Can you work these out from the model? Positions are in its coordinate system, mm. Face numbers are marked on the shaded views. A direction names the side the tool comes from. Coordinates: 2 decimals unless noted, no trailing zeros. Write each loop counter-clockwise with the first axis right and the second up, starting at its lowest first coordinate (ties: lowest second). Pieces come first, ordered by that corner, then holes.
Autodesk Inventor part; units mm, degrees
ref_plane "Work Plane1" through (13.2035, 0, 0) normal (0, 0, 1) x (-1, 0, 0)
ref_plane "YZ Plane" through (0, 0, 0) normal (1, 0, 0) x (0, 1, 0)
ref_plane "XZ Plane" through (0, 0, 0) normal (0, 1, 0) x (-1, 0, 0)
sketch "Skizze1" plane through (0, 0, 0) normal (1, 0, 0) x (0, 1, 0)
  line L0 (2.3094, -4) -> (-2.3094, -4)
  line L1 (-2.3094, -4) -> (-4.6188, 0)
  line L2 (-4.6188, 0) -> (-2.3094, 4)
  line L3 (-2.3094, 4) -> (2.3094, 4)
  line L4 (2.3094, 4) -> (4.6188, 0)
  line L5 (4.6188, 0) -> (2.3094, -4)
  point P0 (0, 0)
  point P1 (0, 0)
  dimension "d0" = 9.2376
extrude "Körper" add sketch "Skizze1" along normal blind 2.45
sketch "Skizze2" plane through (2.45, 0, 0) normal (1, 0, 0) x (0, 0, -1)
  circle A0 centre (0, 0) radius 3.45
  dimension "d7" = 6.9
extrude "Ring" add sketch "Skizze2" along normal blind 2.55
sketch "Skizze3" plane through (0, 0, 0) normal (0, 0, 1) x (1, 0, 0)
  line L0 (0, 2.3094) -> (0, 4.6188)
  line L1 (0, 4.6188) -> (2.45, 4.6188)
  line L2 (2.45, 2.3094) -> (2.45, 4.6188)
  line L3 (-0.49, 0) -> (2.94, 0)
  line L4 (0, 3.45) -> (0.6748, 4.6188)
  line L5 (1.7752, 4.6188) -> (2.45, 3.45)
  dimension "d3" = 30
  dimension "d4" = 30
  dimension "d5" = 6.9
  dimension "d6" = 6.9
revolve "Fase1" cut sketch "Skizze3" angle 360 about axis through (-10, 0, 0) along (1, 0, 0)
sketch "Skizze4" plane through (0, 0, 0) normal (-1, 0, 0) x (0, 0, 1)
  line L0 (0, -6.4663) -> (0, 6.4663)
  line L1 (-5.6, 0) -> (5.6, 0)
  point P0 (0, 0)
hole "Gewinde" at (0, 0, 0) direction (1, 0, 0) diameter 4.134 end through all
chamfer "Fase2" distance 0.433 angle 30 1 edges at (0, 0, -2.067) measured on face at (0, 2.9506, -0.3583)
chamfer "Fase3" distance 0.433 angle 30 1 edges at (5, 0, -2.067) measured on face at (5, -0.4401, -2.9356)
ref_plane "Work Plane1" through (13.2035, 0, 0) normal (0, 0, 1) x (-1, 0, 0)
equation "\"d0\" = 1.1547 * SW"
equation "\"d1\" = KOH1"
equation "\"d7\" = SD2"
equation "\"d8\" = KOH - KOH1"
equation "\"d3\" = ANG1"
equation "\"d4\" = ANG2"
equation "\"d5\" = SW0"
equation "\"d6\" = SW01"
equation "\"d10\" = -0.5 * GD1 + 0.5 * NND"
equation "\"d46\" = -0.5 * GD1 + 0.5 * NND"
equation "\"d12\" = -0.5 * GD1 + 0.5 * NND"
equation "\"d47\" = -0.5 * GD1 + 0.5 * NND"
equation "\"ANG1\" = 30deg"
equation "\"ANG2\" = 30deg"
equation "\"NND\" = 5"
equation "\"KOH1\" = 2.45"
equation "\"KOH\" = 5"
equation "\"SW\" = 8"
equation "\"SW0\" = 6.9"
equation "\"SW01\" = SW0"
equation "\"SD2\" = SW0"
equation "\"GUL\" = 0.541266 * PTC"
equation "\"THREADDIA\" = 5"
equation "\"TOA\" = 30deg"
equation "\"PTC\" = 0.8"
equation "\"E0\" = 1.155 * SW"
equation "\"GAL\" = 0.541266 * PTC"
properties part number "ISO 10511 - M5" material "Stahl, weich"
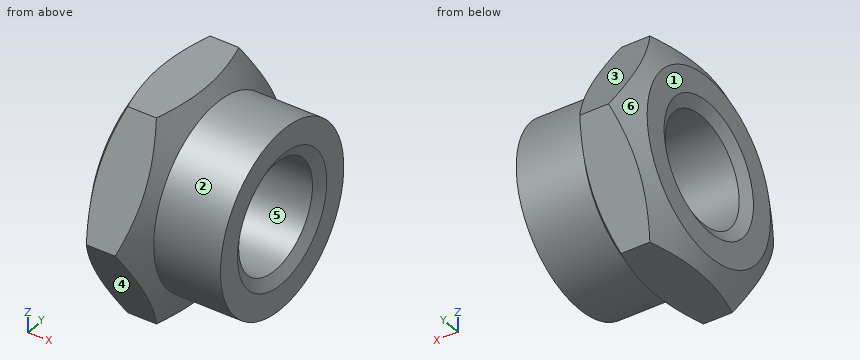
1. Which directions (+Z, -Z, +X, -X, +Y, -Y) give clear straight access to the entire face, cutting with the end or side of a thin tool? Please do the marked faces 1 and 2.
2. If we section it at C-C, the plane x = 2.85: List the corners of the cut face in (y, z) for me, plus the area to 3 significant figures.
3. I'm going to push flat-ended pins straight in: P1, Ø2, axis at y = -3.5, z = 3, coming from the +X side; P2, Ø1.5, axis at x = 1.5, z = -1.5, coming from the +Y side; P3, Ø2, axis at x = 3, z = 2, coming from the +Y side. Where does each tip first touch, or does it pass through?
4. If I drill on L1, parallel to Z at x = 3.8, y = 0; L2, parallel to Z at x = 1.15, y = 0, over which ranges is the centre line in solid material (lowest first)?
5. If we section it at A-A, the plane x = 0.8: List the corners of the cut face in (y, z) for me, plus the area to 3 significant figures.
6. If we section it at B-B, the plane y = 0: List the corners of the cut face in (x, z) for me.
7. We'd pull the mould along Y, two halves only. Please class the marked faces 3, 4, 5 and 6: released by +Y, released by -Y, zero draft, split by the parting line, or undercut.
Answers:
1. face 1: +Z, -Z, -X, +Y, -Y
1. face 2: +X
2. outline: circle Ø6.9 at (0, 0); hole circle Ø4.13 at (0, 0)
2. area: 24.0 mm2
3. P1: stops at x = 2.36
3. P2: stops at y = 4.19
3. P3: stops at y = 3.73
4. L1: z = -3.45 to -2.07, 2.07 to 3.45
4. L2: z = -4 to -2.07, 2.07 to 4
5. outline: (-4.62, 0) - (-2.31, -4) - (2.31, -4) - (4.62, 0) - (2.31, 4) - (-2.31, 4) - close; hole circle Ø4.13 at (0, 0)
5. area: 42.0 mm2
6. outline: (0, -3.45) - (0.32, -4) - (2.13, -4) - (2.45, -3.45) - (5, -3.45) - (5, -2.5) - (4.75, -2.07) - (0.25, -2.07) - (0, -2.5) - close; (0, 2.5) - (0.25, 2.07) - (4.75, 2.07) - (5, 2.5) - (5, 3.45) - (2.45, 3.45) - (2.13, 4) - (0.32, 4) - (0, 3.45) - close
7. face 3: released by +Y
7. face 4: released by -Y
7. face 5: undercut
7. face 6: split by the parting line
